from build123d import *

# Parameters (mm, degrees)
FLANGE_BASE2_DEPTH       = 82.5
CORTE_EXTRUS_O3_START    = -82.5
CORTE_EXTRUS_O3_DEPTH    = 14
CORTE_EXTRUS_O3_START_2  = 68.5
CORTE_EXTRUS_O3_2_DEPTH  = 14
ESBO_O12_W               = 14
ESBO_O12_H               = 1.2
RESSALTO_EXTRUS_O1_DEPTH = 19
FILETE1_R                = 1
ESBO_O13_R               = 4
CORTE_EXTRUS_O4_DEPTH    = 86.316645504


# Read off the part's stored shape, not the designer's step: Corte-extrusão3
# Sheet-metal steps are written as plain solids
with BuildPart() as part:
    # Esboço1 → Flange-base2 (new, symmetric)
    with BuildSketch(Plane(origin=(0, 0, 0), x_dir=(0, 0, -1), z_dir=(1, 0, 0))):
        with BuildLine():
            Line((-18, 9), (-18, 0.7366))
            ThreePointArc((-18, 0.7366), (-17.784254855, 0.215745145), (-17.2634, 0))
            Line((-17.2634, 0), (17.2634, 0))
            ThreePointArc((17.2634, 0), (17.784254855, 0.215745145), (18, 0.7366))
            Line((18, 0.7366), (18, 3))
            Line((18, 3), (19.2, 3))
            Line((19.2, 3), (19.2, 0.7366))
            ThreePointArc((19.2, 0.7366), (18.632782992, -0.632782992), (17.2634, -1.2))
            Line((17.2634, -1.2), (-17.2634, -1.2))
            ThreePointArc((-17.2634, -1.2), (-18.632782992, -0.632782992), (-19.2, 0.7366))
            Line((-19.2, 0.7366), (-19.2, 9))
            Line((-19.2, 9), (-18, 9))
        make_face()
    extrude(amount=FLANGE_BASE2_DEPTH, both=True)

    # Corte-extrusão3 outline → Corte-extrusão3 (cut)
    with BuildSketch(Plane.YZ.offset(CORTE_EXTRUS_O3_START)):
        with BuildLine():
            Line((-1.2, 17.2634), (0, 17.2634))
            ThreePointArc((0, 17.2634), (0.215745145, 17.784254855), (0.7366, 18))
            Line((0.7366, 18), (9, 18))
            Line((9, 18), (9, 19.2))
            Line((9, 19.2), (0.7366, 19.2))
            ThreePointArc((0.7366, 19.2), (-0.632782992, 18.632782992), (-1.2, 17.2634))
        make_face()
        with BuildLine():
            ThreePointArc((0.7366, -18), (0.215745145, -17.784254855), (0, -17.2634))
            Line((0, -17.2634), (-1.2, -17.2634))
            ThreePointArc((-1.2, -17.2634), (-0.632782992, -18.632782992), (0.7366, -19.2))
            Line((0.7366, -19.2), (3, -19.2))
            Line((3, -19.2), (3, -18))
            Line((3, -18), (0.7366, -18))
        make_face()
    extrude(amount=CORTE_EXTRUS_O3_DEPTH, mode=Mode.SUBTRACT)

    # Corte-extrus_o3 2 outline → Corte-extrus_o3 2 (cut)
    with BuildSketch(Plane.YZ.offset(CORTE_EXTRUS_O3_START_2)):
        with BuildLine():
            Line((-1.2, 17.2634), (0, 17.2634))
            ThreePointArc((0, 17.2634), (0.215745145, 17.784254855), (0.7366, 18))
            Line((0.7366, 18), (9, 18))
            Line((9, 18), (9, 19.2))
            Line((9, 19.2), (0.7366, 19.2))
            ThreePointArc((0.7366, 19.2), (-0.632782992, 18.632782992), (-1.2, 17.2634))
        make_face()
        with BuildLine():
            ThreePointArc((0.7366, -18), (0.215745145, -17.784254855), (0, -17.2634))
            Line((0, -17.2634), (-1.2, -17.2634))
            ThreePointArc((-1.2, -17.2634), (-0.632782992, -18.632782992), (0.7366, -19.2))
            Line((0.7366, -19.2), (3, -19.2))
            Line((3, -19.2), (3, -18))
            Line((3, -18), (0.7366, -18))
        make_face()
    extrude(amount=CORTE_EXTRUS_O3_2_DEPTH, mode=Mode.SUBTRACT)

    # Esboço12 → Ressalto-extrusão1 (add, symmetric)
    with BuildSketch(Plane.XY):
        with Locations((75.5, -0.6)):
            Rectangle(ESBO_O12_W, ESBO_O12_H)
        with Locations((-75.5, -0.6)):
            Rectangle(ESBO_O12_W, ESBO_O12_H)
    extrude(amount=RESSALTO_EXTRUS_O1_DEPTH, both=True)

    # Filete1
    filete1_edges = [part.edges().sort_by_distance(p)[0] for p in [
        (82.5, -0.6, -19),
        (82.5, -0.6, 19),
        (-82.5, -0.6, -19),
        (-82.5, -0.6, 19),
    ]]
    fillet(filete1_edges, radius=FILETE1_R)

    # Esboço13 → Corte-extrusão4 (cut, through all)
    with BuildSketch(Plane.XZ.offset(1.2)):
        with Locations(Location((-62.5, 0, 0), (0, 0, 270))):
            Circle(ESBO_O13_R)
    extrude(amount=-CORTE_EXTRUS_O4_DEPTH, mode=Mode.SUBTRACT)


solid = part.part
Geometry: final body of the model. Coordinates: model frame, mm. Coordinates: 2 decimals unless noted, no trailing zeros. Order: outer loops, then holes, each group sorted by start corner. A loop starts at its lowest first (then second) coordinate and runs counter-clockwise, first axis right, second up.
(1) Draft query along Z for faces 1 (the face through (1, 5, 19.2)), 2 (the face through (-66.405, -0.608, 0.867)), 3 (the face through (-1, -1.2, 0)). Return one class per face: pulls with the +Z half, pulls with the -Z half, needs draft (parallel to the pull), parting line crosses it, or undercut.
(2) Section query C-C (z = -13). Return the cut outline in (x, y), plus the area to 3 significant figures.
(3) Material intervals for probe 1 along X at (y, z) = (-0.85, 0); probe 2 along Z at (x, y) = (-35, 1); probe 3 along Z at (x, y) = (13, 5), sorted ascending.
(4) Section query B-B (x = -62.5). Return the cut outline in (y, z), plus the area to 3 significant figures.
(5) Section query A-A (z = 0). Return the cut outline in (x, y).
(6) First-contact query: pin 1 (4 mm diameter, centred on x = -22.5, y = 6.5, fed in from -Z); pin 2 (12 mm diameter, centred on x = 42.5, z = 9, fed in from +Y); pin 3 (1.5 mm diameter, centred on y = 3.5, z = 18.5, fed in from +X); pin 4 (7 mm diameter, centred on x = -62.5, z = 0, fed in from -Y). Flat tips, straight axial feed; report the tip coordinate or a pass-through.
Solution:
1. face 1: pulls with the +Z half
1. face 2: undercut
1. face 3: needs draft
2. outline: (-82.5, -1.2) - (82.5, -1.2) - (82.5, 0) - (-82.5, 0) - close
2. area: 198 mm2
3. probe 1: x = -82.5 to -66.5, -58.5 to 82.5
3. probe 2: z = -19.2 to -18, 18 to 19.2
3. probe 3: z = 18 to 19.2
4. outline: (-1.2, -17.26) arc R1.94 ccw to (0.74, -19.2) - (3, -19.2) - (3, -18) - (0.74, -18) arc R0.74 cw to (0, -17.26) - (0, -4) - (-1.2, -4) - close; (-1.2, 4) - (0, 4) - (0, 17.26) arc R0.74 cw to (0.74, 18) - (9, 18) - (9, 19.2) - (0.74, 19.2) arc R1.94 ccw to (-1.2, 17.26) - close
4. area: 49.5 mm2
5. outline: (-82.5, -1.2) - (-66.5, -1.2) - (-66.5, 0) - (-82.5, 0) - close; (-58.5, -1.2) - (82.5, -1.2) - (82.5, 0) - (-58.5, 0) - close
6. pin 1: stops at z = 18
6. pin 2: stops at y = 0
6. pin 3: stops at x = 68.5
6. pin 4: passes through
